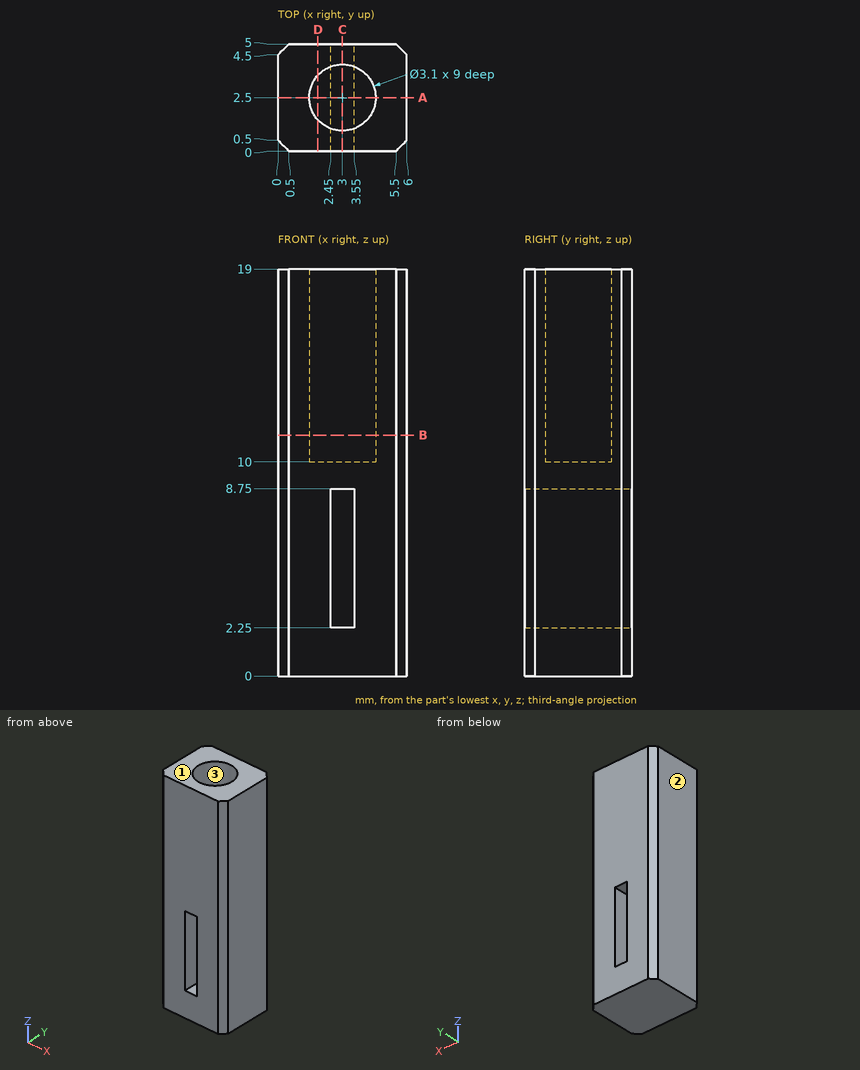
The figure shows three views and two pictorial views of one solid part (mm, origin at its lowest corner). Answer the questions. Give positions to 0.01 mm unless a question says otherwise; leave off trailing zeros. Order: outer loops, then holes, each group sorted by start corner. A loop starts at its lowest first (then second) coordinate and runs counter-clockwise, first axis right, second up. Notation, with made-up numbers: (-38, 1) -> (18, 1) arc R11 cw to (18, 11) -> close; hole circle Ø9 at (76.25, 10.25). An arc over 180 degrees is marked (long way). One line per item, written item: value.
1) Find section C-C, the plane x = 3. Determine the outline of the cut face in (y, z).
Reported:
outline: (0, 0) -> (5, 0) -> (5, 2.25) -> (0, 2.25) -> close; (0, 8.75) -> (5, 8.75) -> (5, 19) -> (4.05, 19) -> (4.05, 10) -> (0.95, 10) -> (0.95, 19) -> (0, 19) -> close
2) Find section D-D, the plane x = 1.85. Determine the outline of the cut face in (y, z).
Reported:
outline: (0, 0) -> (5, 0) -> (5, 19) -> (3.54, 19) -> (3.54, 10) -> (1.46, 10) -> (1.46, 19) -> (0, 19) -> close
3) Find section A-A, the plane y = 2.5. Determine the outline of the cut face in (x, z).
Reported:
outline: (0, 0) -> (6, 0) -> (6, 19) -> (4.55, 19) -> (4.55, 10) -> (1.45, 10) -> (1.45, 19) -> (0, 19) -> close; hole (2.45, 2.25) -> (3.55, 2.25) -> (3.55, 8.75) -> (2.45, 8.75) -> close
4) Determine the mould class of the marked faces 1, 2 and 3 for opening direction X: pulls with the +X half, pulls with the -X half, needs draft (parallel to the pull), parting line crosses it, or undercut.
Reported:
face 1: needs draft
face 2: pulls with the -X half
face 3: undercut
5) A flat-ended cylindrical pin translates along its axis: P1, Ø1, axis at x = 4, y = 2.5, coming from the +Z side. Find the tip coordinate at first contact, or state that the pin passes through.
Reported:
P1: stops at z = 10
6) Find section B-B, the plane z = 11.25. Determine the outline of the cut face in (x, y).
Reported:
outline: (0, 0.5) -> (0.5, 0) -> (5.5, 0) -> (6, 0.5) -> (6, 4.5) -> (5.5, 5) -> (0.5, 5) -> (0, 4.5) -> close; hole circle Ø3.1 at (3, 2.5)
7) Find the intervals of material crossed by line 1 (Y direction, x = 3, z = 13.5); line 2 (X direction, y = 2.5, z = 12.75); line 3 (X direction, y = 0.8, z = 7.75), in increasing order.
Reported:
line 1: y = 0 to 0.95, 4.05 to 5
line 2: x = 0 to 1.45, 4.55 to 6
line 3: x = 0 to 2.45, 3.55 to 6
